```python
from build123d import *

# Parameters (mm, degrees)
F0_W           = 38.5
F0_H           = 55
F0_R           = 2.6
F1_DEPTH       = 5
F2_D           = 2.5
F2_CBORE_D     = 4.5
F2_CBORE_DEPTH = 2.5


with BuildPart() as f1:
    # F0 (on Front) → F1 (new body)
    with BuildSketch(Plane.XZ):
        with Locations((19.25, 27.5)):
            Rectangle(F0_W, F0_H)
        with Locations((19.25, 27.5)):
            Circle(F0_R, mode=Mode.SUBTRACT)
    extrude(amount=-F1_DEPTH)

    # F2 (through all)
    with Locations(Plane.XZ):
        with Locations((3.3, 3.55), (35.2, 3.55), (35.2, 51.45), (3.3, 51.45)):
            CounterBoreHole(F2_D / 2, F2_CBORE_D / 2, F2_CBORE_DEPTH)


solid = f1.part
```
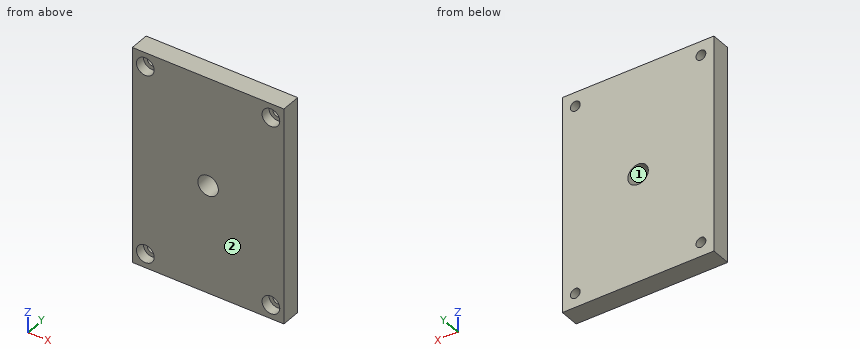
Verification items for the finished model (mm, model axes). Face numbers are marked on the shaded views. Round coordinates to 2 decimals unless told otherwise and drop trailing zeros. Order: outer loops, then holes, each group sorted by start corner. A loop starts at its lowest first (then second) coordinate and runs counter-clockwise, first axis right, second up.
1) Cross-section at A-A, the plane x = 19.25. Record the cut outline in (y, z), plus the area to 3 significant figures.
Geometry says:
outline: (0, 0) - (5, 0) - (5, 24.9) - (0, 24.9) - close; (0, 30.1) - (5, 30.1) - (5, 55) - (0, 55) - close
area: 249 mm2
2) Cross-section at D-D, the plane y = 3.5. Record the cut outline in (x, z).
Geometry says:
outline: (0, 0) - (38.5, 0) - (38.5, 55) - (0, 55) - close; hole circle Ø2.5 at (3.3, 3.55); hole circle Ø2.5 at (3.3, 51.45); hole circle Ø5.2 at (19.25, 27.5); hole circle Ø2.5 at (35.2, 3.55); hole circle Ø2.5 at (35.2, 51.45)
3) Draft check along X on the marked faces 1 and 2. Enter one of: +X half, -X half, draft (parallel to the pull), parting line (faces both ways), or undercut.
Geometry says:
face 1: undercut
face 2: draft
4) Cross-section at C-C, the plane x = 35.2. Record the cut outline in (y, z).
Geometry says:
outline: (0, 0) - (5, 0) - (5, 2.3) - (2.5, 2.3) - (2.5, 1.3) - (0, 1.3) - close; (0, 5.8) - (2.5, 5.8) - (2.5, 4.8) - (5, 4.8) - (5, 50.2) - (2.5, 50.2) - (2.5, 49.2) - (0, 49.2) - close; (0, 53.7) - (2.5, 53.7) - (2.5, 52.7) - (5, 52.7) - (5, 55) - (0, 55) - close
5) Depth check by flat-ended pin: pin 1 (4 mm diameter, centred on x = 35.2, z = 51.45, fed in from -Y). Enter the tip coordinate at first touch or a pass-through.
Geometry says:
pin 1: stops at y = 2.5
6) Cross-section at B-B, the plane z = 27.5. Record the cut outline in (x, y).
Geometry says:
outline: (0, 0) - (16.65, 0) - (16.65, 5) - (0, 5) - close; (21.85, 0) - (38.5, 0) - (38.5, 5) - (21.85, 5) - close
7) Material ranges on line 1 (Z direction, x = 35.2, y = 1.55); line 2 (Z direction, x = 3.3, y = 3.25); line 3 (Z direction, x = 19.25, y = 3.5), recorded low to high.
Geometry says:
line 1: z = 0 to 1.3, 5.8 to 49.2, 53.7 to 55
line 2: z = 0 to 2.3, 4.8 to 50.2, 52.7 to 55
line 3: z = 0 to 24.9, 30.1 to 55
